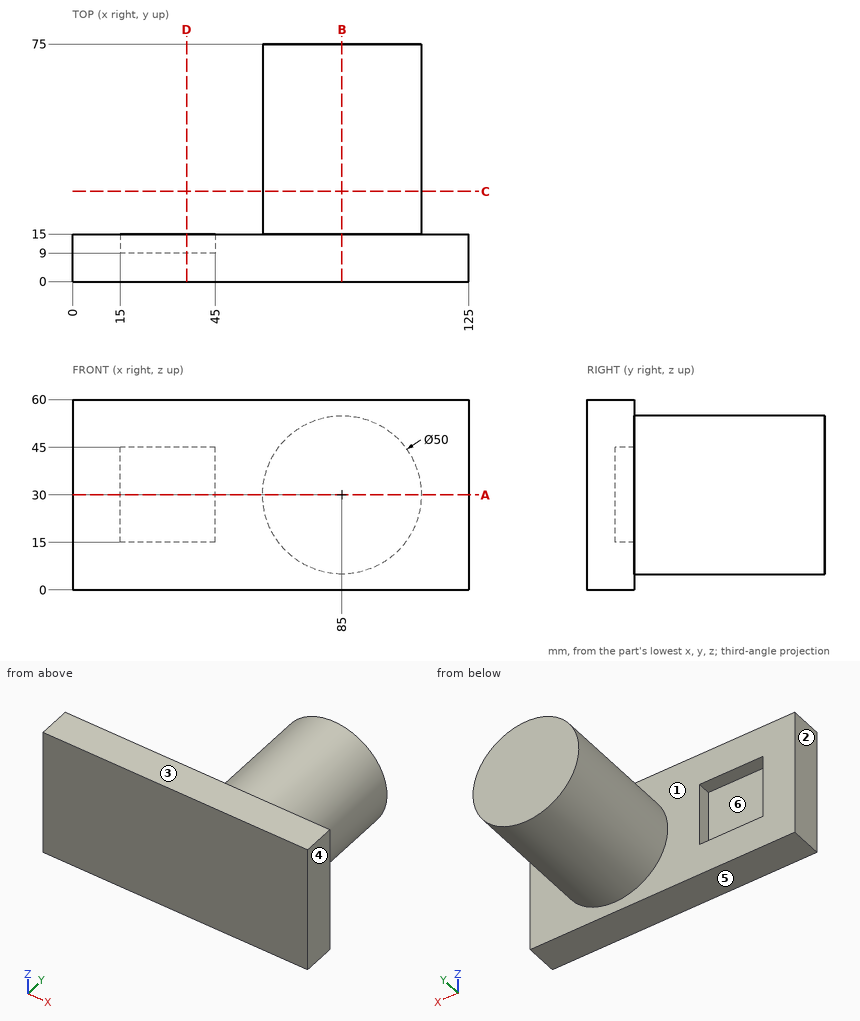
Verification items for this drawing (mm, ordinates from the low corner). A direction names the side the tool comes from. Coordinates: 2 decimals unless noted, no trailing zeros. Order: outer loops, then holes, each group sorted by start corner. A loop starts at its lowest first (then second) coordinate and runs counter-clockwise, first axis right, second up. Notation, with made-up numbers: (15, -10.5) -> (74, -10.5) arc R31 ccw to (74, 15.5) -> close; hole circle Ø2 at (77, 79.5). An arc over 180 degrees is marked (long way). Answer as CSV lines item,"result". Start each with the question number.
1) Cross-section at D-D, the plane x = 36. Record the boundary of the cut face in (y, z).
2) Gauge pin test, flat ends, axial feed: pin 1 Ø12 at (x, y) = (111.5, 30.5) entering from +Z; pin 2 Ø4 at (x, y) = (69, 35) entering from -Z. Record the tip position at first contact, or that the pin passes through.
3) Set-up check for the marked faces 1 and 2: record each of +Z, -Z, +X, -X, +Y, -Y from which the full face is reachable in a straight line by a thin tool's end or side.
4) Release check for a two-part mould opening along Z. For the marked faces 3, 4, 5 and 6 record: released by +Z, released by -Z, zero draft, split by the parting line, or undercut.
5) Cross-section at C-C, the plane y = 28.5. Record the boundary of the cut face in (x, z).
6) Material ranges on L1, parallel to Y at x = 29.5, z = 36.5; L2, parallel to Y at x = 52.5, z = 8; L3, parallel to Z at x = 65, y = 17, recorded low to high. Write a range as [from, to].
7) Cross-section at B-B, the plane x = 85. Record the boundary of the cut face in (y, z).
8) Cross-section at A-A, the plane z = 30. Record the boundary of the cut face in (x, y), then the cut area to 4 significant figures.
Conclusion:
1,outline,"(0, 0) -> (15, 0) -> (15, 15) -> (9, 15) -> (9, 45) -> (15, 45) -> (15, 60) -> (0, 60) -> close"
2,pin 1,"stops at z = 44.31"
2,pin 2,"stops at z = 9.29"
3,face 1,"+Y"
3,face 2,"+Z, -Z, -X, +Y, -Y"
4,face 3,"released by +Z"
4,face 4,"zero draft"
4,face 5,"released by -Z"
4,face 6,"undercut"
5,outline,"circle Ø50 at (85, 30)"
6,L1,"y = [0, 9]"
6,L2,"y = [0, 15]"
6,L3,"z = [15, 45]"
7,outline,"(0, 0) -> (15, 0) -> (15, 5) -> (75, 5) -> (75, 55) -> (15, 55) -> (15, 60) -> (0, 60) -> close"
8,outline,"(0, 0) -> (125, 0) -> (125, 15) -> (110, 15) -> (110, 75) -> (60, 75) -> (60, 15) -> (45, 15) -> (45, 9) -> (15, 9) -> (15, 15) -> (0, 15) -> close"
8,area,"4,695 mm²"
